Part model, mm, in its own coordinate system. Face numbers are marked on the shaded views. A direction names the side the tool comes from. Round coordinates to 2 decimals unless told otherwise and drop trailing zeros. Write each loop counter-clockwise with the first axis right and the second up, starting at its lowest first coordinate (ties: lowest second). Pieces come first, ordered by that corner, then holes. Notation, with made-up numbers: M -8,3 L 14,3 A18 cw 14,34 Z; hole C -22.5,-26.75 d8. An arc over 180 degrees is marked long. Use a Markdown table: item, result. Add a question column.
1) Slice it at C-C on x = 795.75. Write the cut outline in (y, z).
2) Slice it at B-B on y = 460. Write the cut outline in (x, z), plus the area to 3 significant figures.
3) Slice it at A-A on x = 780.5. Write the cut outline in (y, z).
4) Slice it at D-D on z = 5.25. Give the number of separate pieces and of enclosed holes in the cut face, plus the area to 3 significant figures.
5) Wall check: probe 1 along Y at (x, z) = (785.75, 3.25); probe 2 along Y at (x, z) = (789, 4.95); probe 3 along X at (y, z) = (439, 0.9). Give the ranges that are in metal, low to high.
6) Two-plate mould, pull along Y, no slides. Class the marked faces 1, 2 and 3: released by +Y, released by -Y, zero draft, split by the parting line, or undercut.
7) Drop flat-ended pins along their axis: P1, Ø1.7, axis at y = 468, z = 2.5, coming from the -X side; P2, Ø1.7, axis at y = 469, z = 2.5, coming from the +X side; P3, Ø3, axis at y = 455, z = 3, coming from the -X side; P4, Ø1.5, axis at x = 787.66, y = 487.84, coming from the -Z side. Give the stop position or say it passes through.
8) Which spindle directions (+Z, -Z, +X, -X, +Y, -Y) get a long thin tool onto all of the face, cutting with end or side? Do the marked faces 4, 5 and 6. Say none if no direction does.
```python
from build123d import *

# Parameters (mm, degrees)
SKETCH1_R           = 1.25
SKETCH1_R_2         = 1.625
SKETCH1_RX          = 8.302080555
SKETCH1_RY          = 4.346497416
BOSS_EXTRUDE1_DEPTH = 5.85


with BuildPart() as part:
    # Sketch1 → Boss-Extrude1 (new body)
    with BuildSketch(Plane.XY):
        with BuildLine():
            Line((781.409168709, 465.402542), (778.709168709, 465.402542))
            Line((778.709168709, 465.402542), (778.709168709, 461.402176393))
            Line((778.709168709, 461.402176393), (781.409168709, 461.402176393))
            Line((781.409168709, 461.402176393), (781.409168709, 455.752176393))
            Line((781.409168709, 455.752176393), (778.709168709, 455.752176393))
            Line((778.709168709, 455.752176393), (782.620179881, 438.967359197))
            ThreePointArc((782.620179881, 438.967359197), (787.659168709, 434.967516139), (792.698157537, 438.967359197))
            Line((792.698157537, 438.967359197), (796.609168709, 455.752176393))
            Line((796.609168709, 455.752176393), (793.909168709, 455.752176393))
            Line((793.909168709, 455.752176393), (793.909168709, 461.402176393))
            Line((793.909168709, 461.402176393), (796.609168709, 461.402176393))
            Line((796.609168709, 461.402176393), (796.609168709, 465.402542))
            Line((796.609168709, 465.402542), (793.909168709, 465.402542))
            Line((793.909168709, 465.402542), (793.909168709, 471.052542))
            Line((793.909168709, 471.052542), (796.609168709, 471.052542))
            Line((796.609168709, 471.052542), (792.698157537, 487.837359197))
            ThreePointArc((792.698157537, 487.837359197), (787.659168709, 491.837202254), (782.620179881, 487.837359197))
            Line((782.620179881, 487.837359197), (778.709168709, 471.052542))
            Line((778.709168709, 471.052542), (781.409168709, 471.052542))
            Line((781.409168709, 471.052542), (781.409168709, 465.402542))
        make_face()
        with Locations((787.659168709, 487.837359197)):
            Circle(SKETCH1_R, mode=Mode.SUBTRACT)
        with Locations((787.659168709, 438.967359197)):
            Circle(SKETCH1_R, mode=Mode.SUBTRACT)
        with Locations((787.659168709, 463.402359197)):
            Circle(SKETCH1_R_2, mode=Mode.SUBTRACT)
        with Locations(Location((787.659168709, 475.998301041), (0, 0, -90))):
            Ellipse(SKETCH1_RX, SKETCH1_RY, mode=Mode.SUBTRACT)
        with Locations(Location((787.659168709, 450.806417352), (0, 0, -90))):
            Ellipse(SKETCH1_RX, SKETCH1_RY, mode=Mode.SUBTRACT)
    extrude(amount=BOSS_EXTRUDE1_DEPTH)


solid = part.part
```
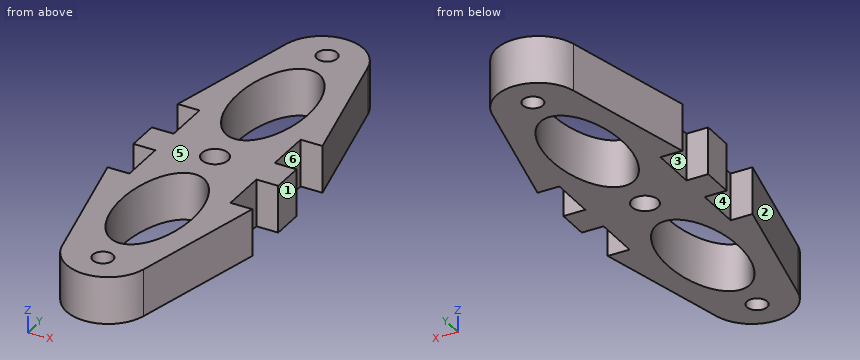
Entries:
| question | item | result |
|---|---|---|
| 1 | outline | M 452.06,0 L 455.75,0 L 455.75,5.85 L 452.06,5.85 Z; M 461.4,0 L 465.4,0 L 465.4,5.85 L 461.4,5.85 Z; M 471.05,0 L 474.74,0 L 474.74,5.85 L 471.05,5.85 Z |
| 2 | outline | M 781.41,0 L 793.91,0 L 793.91,5.85 L 781.41,5.85 Z |
| 2 | area | 73.1 mm^2 |
| 3 | outline | M 448.07,0 L 455.75,0 L 455.75,5.85 L 448.07,5.85 Z; M 461.4,0 L 465.4,0 L 465.4,5.85 L 461.4,5.85 Z; M 471.05,0 L 478.74,0 L 478.74,5.85 L 471.05,5.85 Z |
| 4 | separate pieces | 1 |
| 4 | enclosed holes | 5 |
| 4 | area | 498 mm^2 |
| 5 | probe 1 | y = 435.33 to 443.35, 458.26 to 468.54, 483.46 to 491.47 |
| 5 | probe 2 | y = 435.14 to 442.91, 458.7 to 462.48, 464.32 to 468.1, 483.9 to 491.66 |
| 5 | probe 3 | x = 782.61 to 786.41, 788.91 to 792.71 |
| 6 | face 1 | zero draft |
| 6 | face 2 | released by -Y |
| 6 | face 3 | undercut |
| 7 | P1 | stops at x = 781.41 |
| 7 | P2 | stops at x = 793.91 |
| 7 | P3 | stops at x = 778.71 |
| 7 | P4 | passes through |
| 8 | face 4 | +Z, -Z, -X |
| 8 | face 5 | +Z, +X, -X, +Y, -Y |
| 8 | face 6 | +Z, -Z, +X |
